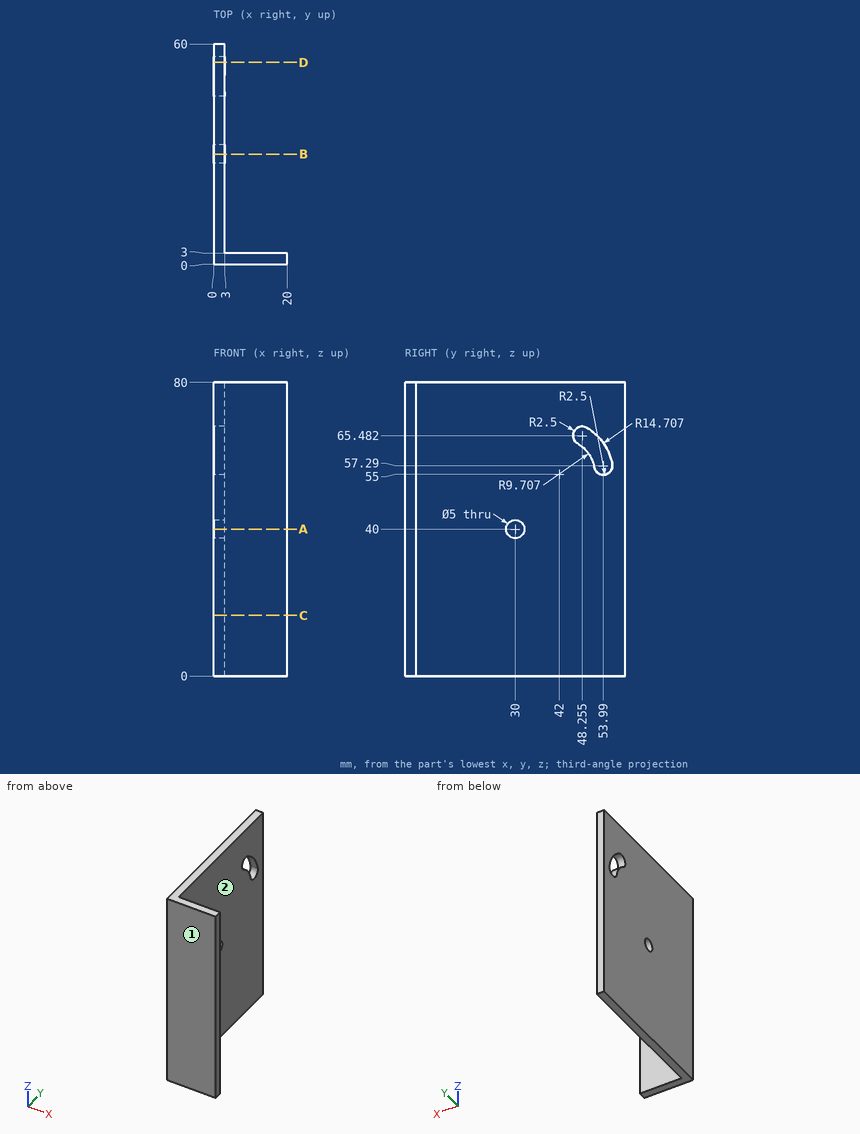
Print and shaded views of the part. All mm, measured from the part's lowest x, y and z. A direction names the side the tool comes from. Coordinates: 2 decimals unless noted, no trailing zeros. Order: outer loops, then holes, each group sorted by start corner. A loop starts at its lowest first (then second) coordinate and runs counter-clockwise, first axis right, second up.
Item 1: Saw through at A-A on z = 40. List the corners of the cut face in (x, y), then the cut area to 3 significant figures.
Filled in:
outline: (0, 0) - (20, 0) - (20, 3) - (3, 3) - (3, 27.5) - (0, 27.5) - close; (0, 32.5) - (3, 32.5) - (3, 60) - (0, 60) - close
area: 216 mm2
Item 2: Saw through at B-B on y = 30. List the corners of the cut face in (x, z).
Filled in:
outline: (0, 0) - (3, 0) - (3, 37.5) - (0, 37.5) - close; (0, 42.5) - (3, 42.5) - (3, 80) - (0, 80) - close
Item 3: Saw through at D-D on y = 55. List the corners of the cut face in (x, z).
Filled in:
outline: (0, 0) - (3, 0) - (3, 55) - (0, 55) - close; (0, 61.88) - (3, 61.88) - (3, 80) - (0, 80) - close
Item 4: Saw through at C-C on z = 16.5. List the corners of the cut face in (x, y).
Filled in:
outline: (0, 0) - (20, 0) - (20, 3) - (3, 3) - (3, 60) - (0, 60) - close
Item 5: Drill centre lines: L1, parallel to Y at x = 2.3, z = 40; L2, parallel to Y at x = 9.5, z = 22. Where is each one in solid material? Low to high.
Filled in:
L1: y = 0 to 27.5, 32.5 to 60
L2: y = 0 to 3
Item 6: Drop flat-ended pins along their axis: pin 1 Ø10 at (x, y) = (9, 22) entering from +Z; pin 2 Ø6 at (y, z) = (26.5, 15) entering from +X. Give the stop position or say it passes through.
Filled in:
pin 1: passes through
pin 2: stops at x = 3
Item 7: Tool access for the marked faces 1 and 2: list every direction of +Z, -Z, +X, -X, +Y, -Y with a clear straight run to the whole face (end or side of a thin tool).
Filled in:
face 1: +Z, -Z, +X, -X, -Y
face 2: +Z, -Z, +X, +Y
